Check sheet for the modelled part. Datum: model origin and axes. Units: mm. Face numbers are marked on the shaded views. A direction names the side the tool comes from. Coordinates: 2 decimals unless noted, no trailing zeros. Loops run counter-clockwise (first coordinate to the right, second up) from the corner with the lowest first, then second, coordinate; pieces in that order, holes last. Notation, with made-up numbers: (84, 74) -> (103, 74) arc R12 cw to (103, 84) -> close; hole circle Ø8 at (-17, -36.75). An arc over 180 degrees is marked (long way). Use CSV: the item, a comma, the result in double quotes.
```python
from build123d import *

# Parameters (mm, degrees)
SKETCH1_W           = 32
SKETCH1_H           = 66
SKETCH1_R           = 1.5
BOSS_EXTRUDE1_DEPTH = 25
SKETCH3_W           = 20
SKETCH3_H           = 55
SKETCH3_H_2         = 1
CUT_EXTRUDE1_DEPTH  = 33
SKETCH4_R           = 6.1
CUT_EXTRUDE6_DEPTH  = 12
SKETCH5_R           = 8.1
CUT_EXTRUDE7_DEPTH  = 5.3
SKETCH7_R           = 1.6
CUT_EXTRUDE8_DEPTH  = 26
CUT_EXTRUDE9_DEPTH  = 10
SKETCH10_W          = 32
SKETCH10_H          = 10
CUT_EXTRUDE10_DEPTH = 10


with BuildPart() as part:
    # Sketch1 → Boss-Extrude1 (new body)
    with BuildSketch(Plane.XY):
        with Locations((16, -33)):
            Rectangle(SKETCH1_W, SKETCH1_H)
        with Locations((16, -4)):
            Circle(SKETCH1_R, mode=Mode.SUBTRACT)
        with Locations((6, -40)):
            Circle(SKETCH1_R, mode=Mode.SUBTRACT)
        with Locations((26, -40)):
            Circle(SKETCH1_R, mode=Mode.SUBTRACT)
    extrude(amount=BOSS_EXTRUDE1_DEPTH)

    # Sketch3 → Cut-Extrude1 (cut, through all)
    with BuildSketch(Plane.ZY):
        with Locations((15, -27.5)):
            Rectangle(SKETCH3_W, SKETCH3_H)
        with Locations((15, -65.5)):
            Rectangle(SKETCH3_W, SKETCH3_H_2)
    extrude(amount=-CUT_EXTRUDE1_DEPTH, mode=Mode.SUBTRACT)

    # Sketch4 → Cut-Extrude6 (cut, through all)
    with BuildSketch(Plane(origin=(0, -55, 0), x_dir=(1, 0, 0), z_dir=(0, 1, 0))):
        with Locations((15.999687497, -15.1)):
            Circle(SKETCH4_R)
    extrude(amount=-CUT_EXTRUDE6_DEPTH, mode=Mode.SUBTRACT)

    # Sketch5 → Cut-Extrude7 (cut)
    with BuildSketch(Plane(origin=(0, -55, 0), x_dir=(1, 0, 0), z_dir=(0, 1, 0))):
        with Locations((15.999687497, -15.1)):
            Circle(SKETCH5_R)
    extrude(amount=-CUT_EXTRUDE7_DEPTH, mode=Mode.SUBTRACT)

    # Sketch7 → Cut-Extrude8 (cut, through all)
    with BuildSketch(Plane.XY.offset(25)):
        with Locations((3.5, -60)):
            Circle(SKETCH7_R)
        with Locations((28.5, -60)):
            Circle(SKETCH7_R)
    extrude(amount=-CUT_EXTRUDE8_DEPTH, mode=Mode.SUBTRACT)

    # Sketch9 → Cut-Extrude9 (cut)
    with BuildSketch(Plane(origin=(0, 0, 0), x_dir=(-1, 0, 0), z_dir=(0, 0, -1))):
        Polygon((-27.219059817, -57.232023799), (-30.256667615, -57.50668516), (-31.537607798, -60.274661361), (-29.780940183, -62.767976201), (-26.743332385, -62.49331484), (-25.462392202, -59.725338639), align=None)
        Polygon((-4.846024949, -57.263082603), (-6.543252468, -59.797233102), (-5.197227519, -62.534150498), (-2.153975051, -62.736917397), (-0.456747532, -60.202766898), (-1.802772481, -57.465849502), align=None)
    extrude(amount=-CUT_EXTRUDE9_DEPTH, mode=Mode.SUBTRACT)

    # Sketch10 → Cut-Extrude10 (cut)
    with BuildSketch(Plane.XY.offset(25)):
        with Locations((16, -60)):
            Rectangle(SKETCH10_W, SKETCH10_H)
    extrude(amount=-CUT_EXTRUDE10_DEPTH, mode=Mode.SUBTRACT)


solid = part.part
```
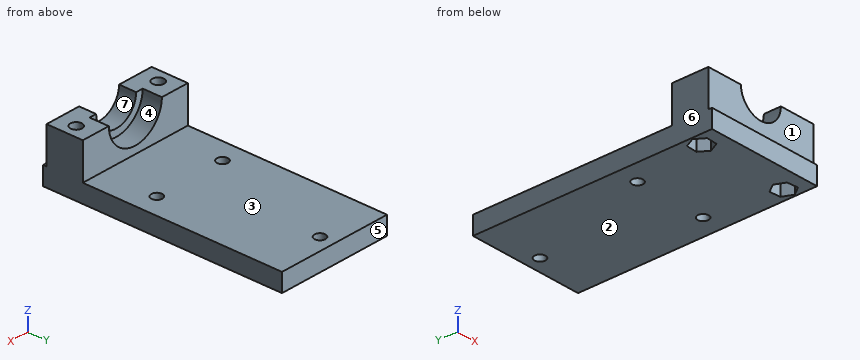
1) Access from +Z, -Z, +X, -X, +Y, -Y to the whole of each face (thin tool, end or side, straight path). Record for the marked faces 1, 2 and 3.
Answer below:
face 1,"+Z, +X, -X, -Y"
face 2,"-Z, +X, -X, +Y, -Y"
face 3,"+Z, +X, -X, +Y"
2) Go/stop test with flat-tipped pins: pin 1 Ø6 at (x, z) = (28.5, 11) entering from -Y; pin 2 Ø8 at (x, z) = (12, 11) entering from +Y; pin 3 Ø16 at (x, y) = (12, -23.5) entering from +Z. Record where each tip stops, or that it passes through.
Answer below:
pin 1,"stops at y = -65"
pin 2,"stops at y = -55"
pin 3,"stops at z = 5"
3) Cross-section at C-C on z = 11.75. Record the boundary of the cut face in (x, y), and give its area (3 significant figures).
Answer below:
outline,"(0, -65) -> (10.9, -65) -> (10.9, -60.3) -> (8.62, -60.3) -> (8.62, -55) -> (0, -55) -> close; (21.1, -65) -> (32, -65) -> (32, -55) -> (23.37, -55) -> (23.37, -60.3) -> (21.1, -60.3) -> close; hole circle Ø3.2 at (3.5, -60); hole circle Ø3.2 at (28.5, -60)"
area,"178 mm²"
4) Cross-section at B-B on x = 16. Record the boundary of the cut face in (y, z).
Answer below:
outline,"(-66, 0) -> (-5.5, 0) -> (-5.5, 5) -> (-55, 5) -> (-55, 7) -> (-60.3, 7) -> (-60.3, 9) -> (-65, 9) -> (-65, 5) -> (-66, 5) -> close; (-2.5, 0) -> (0, 0) -> (0, 5) -> (-2.5, 5) -> close"
5) Thickness scan on line 1 along Y through (x, z) = (16, 2); line 2 along X through (y, z) = (-40, 2.45); line 3 along Y through (x, z) = (28.5, 12.4). Record the ranges inside material, lowest first. Write a range as from..to.
Answer below:
line 1,"y = -66..-5.5, -2.5..0"
line 2,"x = 0..4.5, 7.5..24.5, 27.5..32"
line 3,"y = -65..-61.6, -58.4..-55"
6) Cross-section at D-D on y = -4. Record the boundary of the cut face in (x, z).
Answer below:
outline,"(0, 0) -> (14.5, 0) -> (14.5, 5) -> (0, 5) -> close; (17.5, 0) -> (32, 0) -> (32, 5) -> (17.5, 5) -> close"
7) Draft check along X on the marked faces 4, 5, 6 and 7. Enter one of: released by +X, released by -X, zero draft, split by the parting line, or undercut.
Answer below:
face 4,"undercut"
face 5,"zero draft"
face 6,"released by -X"
face 7,"undercut"
8) Cross-section at A-A on y = -40. Record the boundary of the cut face in (x, z), and give its area (3 significant figures).
Answer below:
outline,"(0, 0) -> (4.5, 0) -> (4.5, 5) -> (0, 5) -> close; (7.5, 0) -> (24.5, 0) -> (24.5, 5) -> (7.5, 5) -> close; (27.5, 0) -> (32, 0) -> (32, 5) -> (27.5, 5) -> close"
area,"130 mm²"
